Geometry: final body of the model. Coordinates: model frame, mm. A direction names the side the tool comes from. Give positions to 0.01 mm unless a question says otherwise; leave off trailing zeros. Write each loop counter-clockwise with the first axis right and the second up, starting at its lowest first coordinate (ties: lowest second). Pieces come first, ordered by that corner, then holes. Notation, with made-up numbers: (40, 17) -> (50, 17) arc R24 cw to (50, 29) -> close; hole circle Ø9 at (23, 22.25). An arc over 180 degrees is marked (long way). Answer in a Markdown table with one row per item. Add a question column.
from build123d import *

# Parameters (mm, degrees)
ESQUISSE1_W              = 106
ESQUISSE1_H              = 332
ESQUISSE1_R              = 3.5
BOSS_EXTRU_1_DEPTH       = 2
ESQUISSE3_R              = 1.375
ENL_V_MAT_EXTRU_1_DEPTH  = 3
CHANFREIN1_SIZE          = 15
CHANFREIN1_SIZE2         = 25.980762114
ESQUISSE4_R              = 1.25
ESQUISSE4_W              = 56
ESQUISSE4_H              = 26
ENL_V_MAT_EXTRU_2_DEPTH  = 10
CONG_1_R                 = 10
ESQUISSE6_R              = 1.25
ESQUISSE6_W              = 20
ESQUISSE6_H              = 2
ESQUISSE6_W_2            = 2
ESQUISSE6_H_2            = 10
ENL_V_MAT_EXTRU_4_DEPTH  = 10
ESQUISSE7_R              = 8
ENL_V_MAT_EXTRU_5_DEPTH  = 10
ESQUISSE8_OUTSIDE_W      = 177.704
ESQUISSE8_OUTSIDE_H      = 403.704
ENL_V_MAT_EXTRU_6_DEPTH  = 10
ESQUISSE10_R             = 1.5
ENL_V_MAT_EXTRU_8_DEPTH  = 10
ESQUISSE11_R             = 1.5
ENL_V_MAT_EXTRU_9_DEPTH  = 10
ENL_V_MAT_EXTRU_10_DEPTH = 10
ESQUISSE13_R             = 8
ENL_V_MAT_EXTRU_11_DEPTH = 10


with BuildPart() as part:
    # Esquisse1 → Boss.-Extru.1 (new body)
    with BuildSketch(Plane(origin=(0, 0, 0), x_dir=(1, 0, 0), z_dir=(0, 1, 0))):
        with Locations((0, 17.5)):
            Rectangle(ESQUISSE1_W, ESQUISSE1_H)
        with Locations((-33, 128.5)):
            Circle(ESQUISSE1_R, mode=Mode.SUBTRACT)
        with Locations((-33, -128.5)):
            Circle(ESQUISSE1_R, mode=Mode.SUBTRACT)
        with Locations((33, 128.5)):
            Circle(ESQUISSE1_R, mode=Mode.SUBTRACT)
        with Locations((33, -128.5)):
            Circle(ESQUISSE1_R, mode=Mode.SUBTRACT)
    extrude(amount=BOSS_EXTRU_1_DEPTH)

    # Esquisse3 → Enlèv. mat.-Extru.1 (cut, through all)
    with BuildSketch(Plane(origin=(0, 2, 0), x_dir=(1, 0, 0), z_dir=(0, 1, 0))):
        with Locations((-22, 11.5)):
            Circle(ESQUISSE3_R)
        with Locations((-22, 97.5)):
            Circle(ESQUISSE3_R)
        with Locations((36, 97.5)):
            Circle(ESQUISSE3_R)
        with Locations((36, 11.5)):
            Circle(ESQUISSE3_R)
    extrude(amount=-ENL_V_MAT_EXTRU_1_DEPTH, mode=Mode.SUBTRACT)

    # Chanfrein1
    chanfrein1_edges = [part.edges().sort_by_distance(p)[0] for p in [
        (-53, 1, -183.5),
        (53, 1, -183.5),
    ]]
    chanfrein1_side = [part.faces().sort_by_distance(p)[0] for p in [
        (0, 1, -183.5),
    ]]
    chamfer(chanfrein1_edges, length=CHANFREIN1_SIZE, length2=CHANFREIN1_SIZE2, reference=chanfrein1_side[0])

    # Esquisse4 → Enlèv. mat.-Extru.2 (cut)
    with BuildSketch(Plane(origin=(0, 2, 0), x_dir=(1, 0, 0), z_dir=(0, 1, 0))):
        with Locations((38, -62.5)):
            Circle(ESQUISSE4_R)
        with Locations((38, -26.5)):
            Circle(ESQUISSE4_R)
        with Locations((-38, -62.5)):
            Circle(ESQUISSE4_R)
        with Locations((-38, -26.5)):
            Circle(ESQUISSE4_R)
        with Locations((0, -44.5)):
            Rectangle(ESQUISSE4_W, ESQUISSE4_H)
    extrude(amount=-ENL_V_MAT_EXTRU_2_DEPTH, mode=Mode.SUBTRACT)

    # Congé1
    cong_1_edges = [part.edges().sort_by_distance(p)[0] for p in [
        (-28, 1, 57.5),
        (-28, 1, 31.5),
        (28, 1, 31.5),
        (28, 1, 57.5),
    ]]
    fillet(cong_1_edges, radius=CONG_1_R)

    # Esquisse6 → Enlèv. mat.-Extru.4 (cut)
    with BuildSketch(Plane(origin=(0, 2, 0), x_dir=(1, 0, 0), z_dir=(0, 1, 0))):
        with Locations((-15, 128.5)):
            Circle(ESQUISSE6_R)
        with Locations((15, 128.5)):
            Circle(ESQUISSE6_R)
        with Locations((-15, 158.5)):
            Circle(ESQUISSE6_R)
        with Locations((15, 158.5)):
            Circle(ESQUISSE6_R)
        with Locations((0, 143.5)):
            Rectangle(ESQUISSE6_W, ESQUISSE6_H)
        with Locations((-0.179881847, 134.5)):
            Rectangle(ESQUISSE6_W_2, ESQUISSE6_H_2)
    extrude(amount=-ENL_V_MAT_EXTRU_4_DEPTH, mode=Mode.SUBTRACT)

    # Esquisse7 → Enlèv. mat.-Extru.5 (cut)
    with BuildSketch(Plane(origin=(0, 2, 0), x_dir=(1, 0, 0), z_dir=(0, 1, 0))):
        with Locations((0, -86.5)):
            Circle(ESQUISSE7_R)
        with Locations((-26.5, -86.5)):
            Circle(ESQUISSE7_R)
    extrude(amount=-ENL_V_MAT_EXTRU_5_DEPTH, mode=Mode.SUBTRACT)

    # Esquisse8 outside → Enlèv. mat.-Extru.6 (cut)
    with BuildSketch(Plane(origin=(0, 2, 0), x_dir=(1, 0, 0), z_dir=(0, 1, 0))):
        with Locations((0, 17.5)):
            Rectangle(ESQUISSE8_OUTSIDE_W, ESQUISSE8_OUTSIDE_H)
        with BuildLine():
            Line((38, 183.5), (-38, 183.5))
            Line((-38, 183.5), (-53, 157.519237886))
            Line((-53, 157.519237886), (-53, -76.5))
            Line((-53, -76.5), (-42.82620953, -130.356234435))
            ThreePointArc((-42.82620953, -130.356234435), (-39.381130607, -136.199426743), (-33, -138.5))
            Line((-33, -138.5), (33, -138.5))
            ThreePointArc((33, -138.5), (39.381130607, -136.199426743), (42.82620953, -130.356234435))
            Line((42.82620953, -130.356234435), (53, -76.5))
            Line((53, -76.5), (53, 157.519237886))
            Line((53, 157.519237886), (38, 183.5))
        make_face(mode=Mode.SUBTRACT)
    extrude(amount=-ENL_V_MAT_EXTRU_6_DEPTH, mode=Mode.SUBTRACT)

    # Esquisse10 → Enlèv. mat.-Extru.8 (cut)
    with BuildSketch(Plane.XZ):
        with Locations((16.063466521, -179.495190528)):
            Circle(ESQUISSE10_R)
        with Locations((41.063466521, -136.193920339)):
            Circle(ESQUISSE10_R)
        with Locations((-41.063466521, -136.193920339)):
            Circle(ESQUISSE10_R)
        with Locations((-16.063466521, -179.495190528)):
            Circle(ESQUISSE10_R)
        Polygon((32.563466521, -150.916352203), (30.18189666, -149.541352203), (26.186846942, -156.460981293), (22.18189666, -163.397758664), (24.563466521, -164.772758664), (29.11009989, -167.397758664), (37.11009989, -153.541352203), align=None)
        Polygon((-24.563466521, -164.772758664), (-22.18189666, -163.397758664), (-26.186846942, -156.460981293), (-30.18189666, -149.541352203), (-32.563466521, -150.916352203), (-37.11009989, -153.541352203), (-29.11009989, -167.397758664), align=None)
    extrude(amount=-ENL_V_MAT_EXTRU_8_DEPTH, mode=Mode.SUBTRACT)

    # Esquisse11 → Enlèv. mat.-Extru.9 (cut)
    with BuildSketch(Plane.XZ):
        with Locations((25, 116)):
            Circle(ESQUISSE11_R)
        with Locations((-25, 116)):
            Circle(ESQUISSE11_R)
    extrude(amount=-ENL_V_MAT_EXTRU_9_DEPTH, mode=Mode.SUBTRACT)

    # Esquisse12 → Enlèv. mat.-Extru.10 (cut)
    with BuildSketch(Plane.XZ):
        with BuildLine():
            Line((38, -31.843333074), (38, -81.843333074))
            ThreePointArc((38, -81.843333074), (33, -86.843333074), (28, -81.843333074))
            Line((28, -81.843333074), (28, -31.843333074))
            ThreePointArc((28, -31.843333074), (33, -26.843333074), (38, -31.843333074))
        make_face()
        with BuildLine():
            Line((18, -31.843333074), (18, -81.843333074))
            ThreePointArc((18, -81.843333074), (13, -86.843333074), (8, -81.843333074))
            Line((8, -81.843333074), (8, -31.843333074))
            ThreePointArc((8, -31.843333074), (13, -26.843333074), (18, -31.843333074))
        make_face()
        with BuildLine():
            Line((-2, -31.843333074), (-2, -81.843333074))
            ThreePointArc((-2, -81.843333074), (-7, -86.843333074), (-12, -81.843333074))
            Line((-12, -81.843333074), (-12, -31.843333074))
            ThreePointArc((-12, -31.843333074), (-7, -26.843333074), (-2, -31.843333074))
        make_face()
        with BuildLine():
            Line((-22, -31.843333074), (-22, -81.843333074))
            ThreePointArc((-22, -81.843333074), (-27, -86.843333074), (-32, -81.843333074))
            Line((-32, -81.843333074), (-32, -31.843333074))
            ThreePointArc((-32, -31.843333074), (-27, -26.843333074), (-22, -31.843333074))
        make_face()
    extrude(amount=-ENL_V_MAT_EXTRU_10_DEPTH, mode=Mode.SUBTRACT)

    # Esquisse13 → Enlèv. mat.-Extru.11 (cut)
    with BuildSketch(Plane.XZ):
        with Locations((0, 6.5)):
            Circle(ESQUISSE13_R)
    extrude(amount=-ENL_V_MAT_EXTRU_11_DEPTH, mode=Mode.SUBTRACT)


solid = part.part
Q1. Access query for faces 1 (the cylindrical face through (-39.5, 1, 136.1)), 2 (the cylindrical face through (-24.99, 0.99, 34.35)). Directions: +Z, -Z, +X, -X, +Y, -Y. A direction counts if a zero-diameter tool reaches every point of the face in a straight line with its end or side. Return the directions, or none.
Q2. Pull-direction query (Z, two-part tool) for faces 3 (the flat face through (-45.605, 0.986, -170.328)), 4 (the flat face through (-1, 2, -25)), 5 (the cylindrical face through (-27.541, 1.014, 78.568)), 6 (the flat face through (47.84, 1.01, 103.81)); classes: +Z half, -Z half, draft (parallel to the pull), parting line (faces both ways), or undercut.
Q3. Section C-C on z = 53. Return loops of the section in (x, y), and give its area (3 significant figures).
Q4. Section B-B on x = 4. Return loops of the section in (y, z).
Q5. Section D-D on y = 0.8. Count the separate pieces of the cut face and the enclosed holes in it, and give its area (3 significant figures).
Q6. Section A-A on z = -77. Return loops of the section in (x, y), and give its area (3 significant figures).
Q7. Line query: probe 1 along X at (y, z) = (0.35, -72.5); probe 2 along X at (y, z) = (1.2, -97.5) (3 decimals); probe 3 along X at (y, z) = (1.5, -128.5). Output: solid intervals per line, ascending. Write a range as from..to.
Checks:
| question | item | result |
|---|---|---|
| 1 | face 1 | +Z, -X, +Y, -Y |
| 1 | face 2 | +Y, -Y |
| 2 | face 3 | -Z half |
| 2 | face 4 | draft |
| 2 | face 5 | undercut |
| 2 | face 6 | +Z half |
| 3 | outline | (-53, 0) -> (-26.35, 0) -> (-26.35, 2) -> (-53, 2) -> close; (26.35, 0) -> (53, 0) -> (53, 2) -> (26.35, 2) -> close |
| 3 | area | 107 mm^2 |
| 4 | outline | (0, -183.5) -> (2, -183.5) -> (2, -144.5) -> (0, -144.5) -> close; (0, -142.5) -> (2, -142.5) -> (2, -0.43) -> (0, -0.43) -> close; (0, 13.43) -> (2, 13.43) -> (2, 31.5) -> (0, 31.5) -> close; (0, 57.5) -> (2, 57.5) -> (2, 79.57) -> (0, 79.57) -> close; (0, 93.43) -> (2, 93.43) -> (2, 138.5) -> (0, 138.5) -> close |
| 5 | separate pieces | 1 |
| 5 | enclosed holes | 34 |
| 5 | area | 28,100 mm^2 |
| 6 | outline | (-53, 0) -> (-32, 0) -> (-32, 2) -> (-53, 2) -> close; (-22, 0) -> (-12, 0) -> (-12, 2) -> (-22, 2) -> close; (-2, 0) -> (8, 0) -> (8, 2) -> (-2, 2) -> close; (18, 0) -> (28, 0) -> (28, 2) -> (18, 2) -> close; (38, 0) -> (53, 0) -> (53, 2) -> (38, 2) -> close |
| 6 | area | 132 mm^2 |
| 7 | probe 1 | -53..-32, -22..-12, -2..8, 18..28, 38..53 |
| 7 | probe 2 | -53..-23.375, -20.625..34.625, 37.375..53 |
| 7 | probe 3 | -53..-36.5, -29.5..-16.25, -13.75..13.75, 16.25..29.5, 36.5..53 |
